from build123d import *

# Parameters (mm, degrees)
BOSS_EXTRUDE1_DEPTH = 3
SKETCH2_R           = 3.5
SKETCH2_R_2         = 2
CUT_EXTRUDE1_DEPTH  = 4


with BuildPart() as part:
    # Sketch1 → Boss-Extrude1 (new body)
    with BuildSketch(Plane(origin=(0, 0, 0), x_dir=(1, 0, 0), z_dir=(0, 1, 0))):
        Polygon((-15, -6), (-15, -15), (15, -15), (15, -6), (25, -6), (25, 6), (15, 6), (15, 15), (-15, 15), (-15, 6), (-25, 6), (-25, -6), align=None)
    extrude(amount=BOSS_EXTRUDE1_DEPTH)

    # Sketch2 → Cut-Extrude1 (cut, through all)
    with BuildSketch(Plane(origin=(0, 3, 0), x_dir=(1, 0, 0), z_dir=(0, 1, 0))):
        with Locations((-20, 0)):
            Circle(SKETCH2_R)
        with Locations((-11.75, 12)):
            Circle(SKETCH2_R_2)
        with Locations((-11.75, -12)):
            Circle(SKETCH2_R_2)
        with Locations((11.75, -12)):
            Circle(SKETCH2_R_2)
        with Locations((20, 0)):
            Circle(SKETCH2_R)
        with Locations((11.75, 12)):
            Circle(SKETCH2_R_2)
    extrude(amount=-CUT_EXTRUDE1_DEPTH, mode=Mode.SUBTRACT)


solid = part.part
Could you check a few things on this model? Use its own coordinates, in mm. A direction names the side the tool comes from. Coordinates: 2 decimals unless noted, no trailing zeros. Write each loop counter-clockwise with the first axis right and the second up, starting at its lowest first coordinate (ties: lowest second). Pieces come first, ordered by that corner, then holes. Notation, with made-up numbers: (-20, -20) - (20, -20) arc R30 cw to (20, 16) - close; hole circle Ø7 at (-16.75, 64). An arc over 180 degrees is marked (long way). Write item = value, one per line.
1) Will these pins go through, and if not, where does the flat tip stop? pin 1 Ø0.9 at (y, z) = (1, -10.5) entering from +X; pin 2 Ø2.5 at (x, z) = (11.75, 12) entering from -Y; pin 3 Ø2 at (x, z) = (-3.5, -6.5) entering from -Y; pin 4 Ø0.9 at (x, y) = (18.5, 1) entering from -Z.
Result set:
pin_1 = 15
pin_2 = through
pin_3 = 0
pin_4 = -6
2) Suppose I cut it at D-D on y = 0.95. Please give me the cut outline in (x, z), plus the area to 3 significant figures.
Result set:
outline = (-25, -6) - (-15, -6) - (-15, -15) - (15, -15) - (15, -6) - (25, -6) - (25, 6) - (15, 6) - (15, 15) - (-15, 15) - (-15, 6) - (-25, 6) - close; hole circle Ø7 at (-20, 0); hole circle Ø4 at (-11.75, -12); hole circle Ø4 at (-11.75, 12); hole circle Ø4 at (11.75, -12); hole circle Ø4 at (11.75, 12); hole circle Ø7 at (20, 0)
area = 1,010 mm2
3) Suppose I cut it at B-B on x = -11.75. Please give me the cut outline in (y, z).
Result set:
outline = (0, -15) - (3, -15) - (3, -14) - (0, -14) - close; (0, -10) - (3, -10) - (3, 10) - (0, 10) - close; (0, 14) - (3, 14) - (3, 15) - (0, 15) - close
4) Suppose I cut it at C-C on x = -20. Please give me the cut outline in (y, z), plus the area to 3 significant figures.
Result set:
outline = (0, -6) - (3, -6) - (3, -3.5) - (0, -3.5) - close; (0, 3.5) - (3, 3.5) - (3, 6) - (0, 6) - close
area = 15.0 mm2
5) Please list where these lines run through material, in increasing order: line 1 (X direction, y = 1.25, z = 0); line 2 (X direction, y = 1.9, z = -12); line 3 (Z direction, x = -11.75, y = 1.7). Write a range as [from, to].
Result set:
line_1 = [-25, -23.5], [-16.5, 16.5], [23.5, 25]
line_2 = [-15, -13.75], [-9.75, 9.75], [13.75, 15]
line_3 = [-15, -14], [-10, 10], [14, 15]
6) We'd pull the mould along X, two halves only. Please class faces 5 (the flat face through (25, 1, 0)), 6 (the flat face through (-15, 1, 10)), 7 (the flat face through (0, 0, 0)), 8 (the cylindrical face through (23.34, 1.52, -1.05)): +X half, -X half, draft (parallel to the pull), parting line (faces both ways), or undercut.
Result set:
face_5 = +X half
face_6 = -X half
face_7 = draft
face_8 = undercut
7) Suppose I cut it at A-A on z = -12. Please give me the cut outline in (x, y), plus the area to 3 significant figures.
Result set:
outline = (-15, 0) - (-13.75, 0) - (-13.75, 3) - (-15, 3) - close; (-9.75, 0) - (9.75, 0) - (9.75, 3) - (-9.75, 3) - close; (13.75, 0) - (15, 0) - (15, 3) - (13.75, 3) - close
area = 66.0 mm2
8) For faces 1 (the flat face through (20, 1, -6)), 2 (the flat face through (-15, 1, -11)), 3 (the flat face through (15, 1, 11)), 4 (the flat face through (-20, 1, 6)), which set-ups out of +Z, -Z, +X, -X, +Y, -Y let a thin tool reach every point of the face, with its end or its side?
Result set:
face_1 = -Z, +X, +Y, -Y
face_2 = -Z, -X, +Y, -Y
face_3 = +Z, +X, +Y, -Y
face_4 = +Z, -X, +Y, -Y
